Build history of the part. All positions in model axes, mm. Face numbers are marked on the shaded views. A direction names the side the tool comes from. Round coordinates to 2 decimals unless told otherwise and drop trailing zeros. Order: outer loops, then holes, each group sorted by start corner. A loop starts at its lowest first (then second) coordinate and runs counter-clockwise, first axis right, second up. Notation, with made-up numbers: M 9,68 L 58,68 A20 cw 58,75 Z; hole C -36,-2.75 d7. An arc over 180 degrees is marked long. Use CSV: the item, a comma, the result in double quotes.
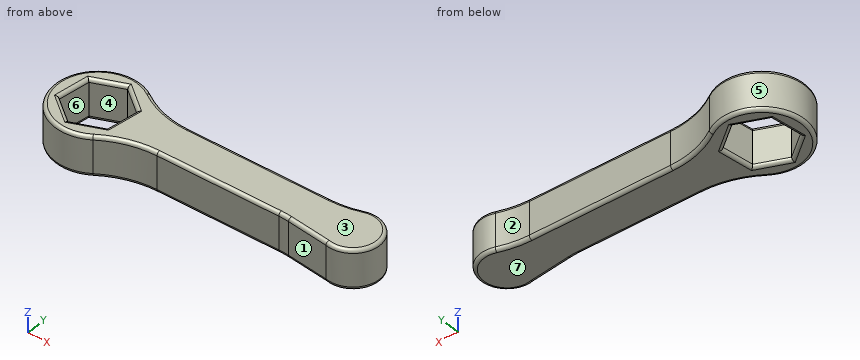
from build123d import *

# Parameters (mm, degrees)
F1_DEPTH    = 6
F2_R        = 14
F3_T1_DEPTH = 6
F4_R        = 13
F5_R        = 0.5


# Not quite as in the source:
# - a fillet or chamfer that OpenCascade refuses, or shapes differently, is made with other operations: its cross-section is extruded or revolved along the edge and cut away or added


with BuildPart() as f1:
    # F0 (on Top) → F1 (new body)
    with BuildSketch(Plane.XY):
        with BuildLine():
            Line((36.1013870801, 3.026675175), (5.7523245202, 3.026675175))
            ThreePointArc((5.7523245202, 3.026675175), (-6.5, 0), (5.7523245202, -3.026675175))
            Line((5.7523245202, -3.026675175), (36.1013870801, -3.026675175))
            ThreePointArc((36.1013870801, -3.026675175), (42.7283578295, 0), (36.1013870801, 3.026675175))
        make_face()
        Polygon((-3.7867383436, 2.9366555893), (0.6498491707, 4.7477393977), (4.4365875143, 1.8110838084), (3.7867383436, -2.9366555893), (-0.6498491707, -4.7477393977), (-4.4365875143, -1.8110838084), align=None, mode=Mode.SUBTRACT)
    extrude(amount=F1_DEPTH)

    # F2
    f2_edges = [f1.edges().sort_by_distance(p)[0] for p in [
        (5.752325, -3.026675, 3),
        (5.752325, 3.026675, 3),
        (36.101387, 3.026675, 3),
    ]]
    fillet(f2_edges, radius=F2_R)

    # F3: chamfer of 11 on 1 edges, made by hand

    # F3_s2 → F3_t1 (join)
    with BuildSketch(Plane.XY):
        with BuildLine():
            Line((30.2515384912, -2.9735152662), (38.1998957411, -3.9409061384))
            Line((38.1998957411, -3.9409061384), (38.2526662364, -3.7273288109))
            ThreePointArc((38.2526662364, -3.7273288109), (37.1662038799, -3.4493250658), (36.2454465167, -2.8604016692))
            Line((36.2454465167, -2.8604016692), (36.1013870801, -2.806675175))
            ThreePointArc((36.1013870801, -2.806675175), (33.1764627857, -2.806675175), (30.2515384912, -2.7535152662))
            Line((30.2515384912, -2.7535152662), (30.2515384912, -2.9735152662))
        make_face()
    extrude(amount=F3_T1_DEPTH)

    # F4
    f4_edges = [f1.edges().sort_by_distance(p)[0] for p in [
        (30.688315, -3.026675, 3),
    ]]
    fillet(f4_edges, radius=F4_R)

    # F5
    f5_edges = [f1.edges().sort_by_distance(p)[0] for p in [
        (20.658434, -3.026675, 0),
        (30.686871, -3.050504, 0),
        (7.341933, -3.632803, 0),
        (34.616932, -3.504825, 0),
        (-6.5, 0, 0),
        (42.724404, 0.177915, 0),
        (7.341933, 3.632803, 0),
        (35.177697, 3.218098, 0),
        (22.143624, 3.026675, 0),
        (-4.111663, 0.562786, 0),
        (-1.568445, 3.842197, 0),
        (2.543218, 3.279412, 0),
        (4.111663, -0.562786, 0),
        (1.568445, -3.842197, 0),
        (-2.543218, -3.279412, 0),
        (20.658434, -3.026675, 6),
        (30.686871, -3.050504, 6),
        (7.341933, -3.632803, 6),
        (34.616932, -3.504825, 6),
        (-6.5, 0, 6),
        (42.724404, 0.177915, 6),
        (7.341933, 3.632803, 6),
        (35.177697, 3.218098, 6),
        (22.143624, 3.026675, 6),
        (-4.111663, 0.562786, 6),
        (-1.568445, 3.842197, 6),
        (2.543218, 3.279412, 6),
        (4.111663, -0.562786, 6),
        (1.568445, -3.842197, 6),
        (-2.543218, -3.279412, 6),
    ]]
    fillet(f5_edges, radius=F5_R)


solid = f1.part
(1) Drop flat-ended pins along their axis: pin 1 (1.5 mm diameter, centred on y = 4.5, z = 3.5, fed in from -X); pin 2 (2.5 mm diameter, centred on x = 23, z = 2, fed in from -Y); pin 3 (2 mm diameter, centred on x = -1.5, z = 1, fed in from -Y). Give the stop position or say it passes through.
Answer block:
pin 1,"stops at x = -5.31"
pin 2,"stops at y = -3.03"
pin 3,"stops at y = -6.48"
(2) Cut at B-B, the plane x = 15. Give the cut face in (y, z), and give its area (3 significant figures).
Answer block:
outline,"M -3.03,0.5 A0.5 ccw -2.53,0 L 2.53,0 A0.5 ccw 3.03,0.5 L 3.03,5.5 A0.5 ccw 2.53,6 L -2.53,6 A0.5 ccw -3.03,5.5 Z"
area,"36.1 mm²"
(3) Cut at A-A, the plane z = 4. Give the cut face in (x, y).
Answer block:
outline,"M 3.62,-5.4 A14 cw 11.42,-3.03 L 29.9,-3.03 A13 cw 31.47,-3.12 L 37.76,-3.89 A4 ccw long 37.42,3.79 A14 cw 32.87,3.03 L 11.42,3.03 A14 cw 3.62,5.4 A6.5 ccw long Z; hole M -4.44,-1.81 L -0.65,-4.75 L 3.79,-2.94 L 4.44,1.81 L 0.65,4.75 L -3.79,2.94 Z"
(4) Wall check: line 1 (Y direction, x = 22, z = 2.25); line 2 (Y direction, x = 39, z = 1); line 3 (X direction, y = -0.25, z = 4). Give the ranges that are in metal, low to high. Write a range as from..to.
Answer block:
line 1,"y = -3.03..3.03"
line 2,"y = -4..4"
line 3,"x = -6.5..-4.22, 4.15..42.72"
(5) Two-plate mould, pull along X, no slides. Class the marked faces 5, 6 and 7: released by +X, released by -X, zero draft, split by the parting line, or undercut.
Answer block:
face 5,"split by the parting line"
face 6,"undercut"
face 7,"zero draft"
(6) Tool access for the marked faces 1, 2, 3 and 4: list every direction of +Z, -Z, +X, -X, +Y, -Y with a clear straight run to the whole face (end or side of a thin tool).
Answer block:
face 1,"+Z, -Z, -Y"
face 2,"+Z, -Z, +Y"
face 3,"+Z, +X, -X, +Y, -Y"
face 4,"+Z, -Z"
